from build123d import *

# Parameters (mm, degrees)
SKETCH_1_R          = 1.65
EXTRUDE_1_DEPTH     = 3
CUT_EXTRUDE_START   = -28
CUT_EXTRUDE_3_DEPTH = 28
FILLET_1_R          = 100


with BuildPart() as part:
    # 草图1 → 凸台-拉伸1 (new body)
    with BuildSketch(Plane.XY):
        with BuildLine():
            Line((0, 0), (20, 0))
            Line((20, 0), (20, 40))
            ThreePointArc((20, 40), (10, 50), (0, 40))
            Line((0, 40), (0, 0))
        make_face()
        with Locations((10, 40)):
            Circle(SKETCH_1_R, mode=Mode.SUBTRACT)
        with Locations((10, 8)):
            Circle(SKETCH_1_R, mode=Mode.SUBTRACT)
        with Locations((10, 23)):
            Circle(SKETCH_1_R, mode=Mode.SUBTRACT)
    extrude(amount=EXTRUDE_1_DEPTH)

    # 草图4 → 切除-拉伸3 (cut)
    with BuildSketch(Plane.XY.offset(3).offset(CUT_EXTRUDE_START)):
        with BuildLine():
            Line((0, 40), (5, 40))
            ThreePointArc((5, 40), (10, 45), (15, 40))
            Line((15, 40), (20, 40))
            ThreePointArc((20, 40), (10, 50), (0, 40))
        make_face()
    extrude(amount=CUT_EXTRUDE_3_DEPTH, mode=Mode.SUBTRACT)

    # 圆角1
    # the kernel refuses this fillet: 100 mm, written as the material it takes off along each edge
    with BuildSketch(Plane(origin=(20, 40, -78.06247498), x_dir=(0, -1, 0), z_dir=(0, 0, 1))) as fillet_1_piece_1:
        with BuildLine():
            CenterArc((31.224989992, -100), FILLET_1_R, 90, 18.194872339)
            Line((0, -5), (0, 0))
            Line((0, 0), (31.224989992, 0))
        make_face()
    extrude(amount=159.12494996, mode=Mode.SUBTRACT)
    with BuildSketch(Plane(origin=(0, 40, -78.06247498), x_dir=(0, -1, 0), z_dir=(0, 0, 1))) as fillet_1_piece_2:
        with BuildLine():
            CenterArc((31.224989992, 100), FILLET_1_R, 251.805127661, 18.194872339)
            Line((0, 5), (0, 0))
            Line((0, 0), (31.224989992, 0))
        make_face()
    extrude(amount=159.12494996, mode=Mode.SUBTRACT)


solid = part.part
Could you check a few things on this model? Use its own coordinates, in mm. Coordinates: 2 decimals unless noted, no trailing zeros. Order: outer loops, then holes, each group sorted by start corner. A loop starts at its lowest first (then second) coordinate and runs counter-clockwise, first axis right, second up. Notation, with made-up numbers: (47, 79) - (78, 79) arc R25 ccw to (78, 108) - close; hole circle Ø3 at (-32.5, 38.25). An arc over 180 degrees is marked (long way). Answer in a Markdown table with one row per item. Add a question column.
(1) I need wall thicknesses on L1, parallel to Y at x = 10, z = 2; L2, parallel to Y at x = 10.75, z = 1.45; L3, parallel to X at y = 6.5, z = 1.7. Which ranges of each line are inside material? Lowest first, please.
(2) If we section it at B-B, the plane x = 10: Please give me the cut outline in (y, z), then the cut area to 3 significant figures.
(3) Will these pins go through, and if not, where does the flat tip stop? pin 1 (1.5 mm diameter, centred on y = 30.5, z = 1, fed in from +X); pin 2 (10 mm diameter, centred on x = 3, y = 18, fed in from -Z); pin 3 (2 mm diameter, centred on x = 10, y = 23, fed in from +Z) (1 decimal).
(4) If we section it at A-A, the plane y = 8: Please give me the cut outline in (x, z).
(5) If we section it at C-C, the plane z = 1.8: Please give me the cut outline in (x, y), then the cut area to 3 significant figures.
(6) If we section it at D-D, the plane y = 23: Please give me the cut outline in (x, z).
(7) If we mould it in two halves opening along X, with no side actions, what happens to faces 1 (the face through (10, 45, 1)), 2 (the face through (9.785, 24.636, 1.479)), 3 (the face through (18.777, 24.367, 1.479)), 4 (the face through (10.89, 9.39, 1.48))? For each: released by +X, released by -X, zero draft, split by the parting line, or undercut.
Results are:
| question | item | result |
|---|---|---|
| 1 | L1 | y = 0 to 6.35, 9.65 to 21.35, 24.65 to 38.35, 41.65 to 45 |
| 1 | L2 | y = 0 to 6.53, 9.47 to 21.53, 24.47 to 38.53, 41.47 to 44.94 |
| 1 | L3 | x = 0 to 9.31, 10.69 to 20 |
| 2 | outline | (0, 0) - (6.35, 0) - (6.35, 3) - (0, 3) - close; (9.65, 0) - (21.35, 0) - (21.35, 3) - (9.65, 3) - close; (24.65, 0) - (38.35, 0) - (38.35, 3) - (24.65, 3) - close; (41.65, 0) - (45, 0) - (45, 3) - (41.65, 3) - close |
| 2 | area | 105 mm2 |
| 3 | pin 1 | stops at x = 17.78 |
| 3 | pin 2 | stops at z = 0 |
| 3 | pin 3 | passes through |
| 4 | outline | (0, 0) - (8.35, 0) - (8.35, 3) - (0, 3) - close; (11.65, 0) - (20, 0) - (20, 3) - (11.65, 3) - close |
| 5 | outline | (0, 0) - (20, 0) - (20, 8.78) arc R100 ccw to (15, 40) arc R5 ccw to (5, 40) arc R100 ccw to (0, 8.78) - close; hole circle Ø3.3 at (10, 8); hole circle Ø3.3 at (10, 23); hole circle Ø3.3 at (10, 40) |
| 5 | area | 711 mm2 |
| 6 | outline | (1.02, 0) - (8.35, 0) - (8.35, 3) - (1.02, 3) - close; (11.65, 0) - (18.98, 0) - (18.98, 3) - (11.65, 3) - close |
| 7 | face 1 | split by the parting line |
| 7 | face 2 | undercut |
| 7 | face 3 | released by +X |
| 7 | face 4 | undercut |
